```python
from build123d import *

# Parameters (mm, degrees)
SKETCH1_W                 = 100
SKETCH1_H                 = 155
BOSS_EXTRUDE1_DEPTH       = 7.5
SKETCH2_R                 = 2.05
SKETCH2_W                 = 60
SKETCH2_H                 = 17.5
HOLE_CUTOUTS_DEPTH        = 8.5
SKETCH3_W                 = 25
SKETCH3_H                 = 2.5
BATTERY_STRAP_HOLES_DEPTH = 8.5
H_BRIDGE_HOLES_DEPTH      = 7.5
FILLET1_R                 = 2
CAMERA_WIRE_HOLE_DEPTH    = 8.5
SKETCH10_R                = 2.05
CUT_EXTRUDE1_DEPTH        = 7.5
SKETCH11_R                = 3
CUT_EXTRUDE2_DEPTH        = 3


with BuildPart() as part:
    # Sketch1 → Boss-Extrude1 (new body)
    with BuildSketch(Plane.XY):
        with Locations((50, 77.5)):
            Rectangle(SKETCH1_W, SKETCH1_H)
    extrude(amount=BOSS_EXTRUDE1_DEPTH)

    # Sketch2 → Hole cutouts (cut, through all)
    with BuildSketch(Plane.XY.offset(7.5)):
        with Locations((10.45, 146.45)):
            Circle(SKETCH2_R)
        with Locations((89.95, 143.95)):
            Circle(SKETCH2_R)
        with Locations((89.95, 11.05)):
            Circle(SKETCH2_R)
        with Locations((10.45, 8.55)):
            Circle(SKETCH2_R)
        with Locations((50.2, 146.25)):
            Rectangle(SKETCH2_W, SKETCH2_H)
        with Locations((50.2, 8.75)):
            Rectangle(SKETCH2_W, SKETCH2_H)
    extrude(amount=-HOLE_CUTOUTS_DEPTH, mode=Mode.SUBTRACT)

    # Sketch3 → Battery strap holes (cut, through all)
    with BuildSketch(Plane.XY.offset(7.5)):
        with Locations((22.5, 89.75)):
            Rectangle(SKETCH3_W, SKETCH3_H)
        with Locations((77.5, 89.75)):
            Rectangle(SKETCH3_W, SKETCH3_H)
        with Locations((22.5, 55.25)):
            Rectangle(SKETCH3_W, SKETCH3_H)
        with Locations((77.5, 55.25)):
            Rectangle(SKETCH3_W, SKETCH3_H)
    extrude(amount=-BATTERY_STRAP_HOLES_DEPTH, mode=Mode.SUBTRACT)

    # Sketch4 → H-Bridge Holes (cut)
    with BuildSketch(Plane.XY.offset(7.5)):
        with BuildLine():
            Line((6, 133.51), (4, 133.51))
            ThreePointArc((4, 133.51), (2.25, 131.76), (4, 130.01))
            Line((4, 130.01), (5, 130.01))
            Line((5, 130.01), (5, 131.76))
            Line((5, 131.76), (7.75, 131.76))
            ThreePointArc((7.75, 131.76), (7.237436867, 132.997436867), (6, 133.51))
        make_face()
        with BuildLine():
            ThreePointArc((6, 130.01), (7.237436867, 130.522563133), (7.75, 131.76))
            Line((7.75, 131.76), (5, 131.76))
            Line((5, 131.76), (5, 130.01))
            Line((5, 130.01), (6, 130.01))
        make_face()
        with BuildLine():
            Line((42.5, 131.76), (39.75, 131.76))
            ThreePointArc((39.75, 131.76), (40.262563133, 130.522563133), (41.5, 130.01))
            Line((41.5, 130.01), (42.5, 130.01))
            Line((42.5, 130.01), (42.5, 131.76))
        make_face()
        with BuildLine():
            ThreePointArc((41.5, 133.51), (40.262563133, 132.997436867), (39.75, 131.76))
            Line((39.75, 131.76), (42.5, 131.76))
            Line((42.5, 131.76), (42.5, 130.01))
            Line((42.5, 130.01), (43.5, 130.01))
            ThreePointArc((43.5, 130.01), (45.25, 131.76), (43.5, 133.51))
            Line((43.5, 133.51), (41.5, 133.51))
        make_face()
        with BuildLine():
            Line((5, 94), (5, 95.75))
            Line((5, 95.75), (4, 95.75))
            ThreePointArc((4, 95.75), (2.25, 94), (4, 92.25))
            Line((4, 92.25), (6, 92.25))
            ThreePointArc((6, 92.25), (7.237436867, 92.762563133), (7.75, 94))
            Line((7.75, 94), (5, 94))
        make_face()
        with BuildLine():
            Line((6, 95.75), (5, 95.75))
            Line((5, 95.75), (5, 94))
            Line((5, 94), (7.75, 94))
            ThreePointArc((7.75, 94), (7.237436867, 95.237436867), (6, 95.75))
        make_face()
        with BuildLine():
            Line((43.5, 95.75), (42.5, 95.75))
            Line((42.5, 95.75), (42.5, 94))
            Line((42.5, 94), (39.75, 94))
            ThreePointArc((39.75, 94), (40.262563133, 92.762563133), (41.5, 92.25))
            Line((41.5, 92.25), (43.5, 92.25))
            ThreePointArc((43.5, 92.25), (45.25, 94), (43.5, 95.75))
        make_face()
        with BuildLine():
            Line((42.5, 94), (42.5, 95.75))
            Line((42.5, 95.75), (41.5, 95.75))
            ThreePointArc((41.5, 95.75), (40.262563133, 95.237436867), (39.75, 94))
            Line((39.75, 94), (42.5, 94))
        make_face()
    extrude(amount=-H_BRIDGE_HOLES_DEPTH, mode=Mode.SUBTRACT)

    # Fillet1
    fillet1_edges = [part.edges().sort_by_distance(p)[0] for p in [
        (20.2, 0, 3.75),
        (20.2, 17.5, 3.75),
        (80.2, 17.5, 3.75),
        (80.2, 0, 3.75),
        (20.2, 137.5, 3.75),
        (20.2, 155, 3.75),
        (80.2, 155, 3.75),
        (80.2, 137.5, 3.75),
        (0, 155, 3.75),
        (100, 155, 3.75),
        (100, 0, 3.75),
        (0, 0, 3.75),
    ]]
    fillet(fillet1_edges, radius=FILLET1_R)

    # Sketch9 → Camera Wire Hole (cut, through all)
    with BuildSketch(Plane.XY.offset(7.5)):
        with BuildLine():
            Line((0, 82.5), (0, 62.5))
            ThreePointArc((0, 62.5), (10, 72.5), (0, 82.5))
        make_face()
    extrude(amount=-CAMERA_WIRE_HOLE_DEPTH, mode=Mode.SUBTRACT)

    # Sketch10 → Cut-Extrude1 (cut)
    with BuildSketch(Plane.XY.offset(7.5)):
        with Locations((3.8, 4.55)):
            Circle(SKETCH10_R)
        with Locations((95.025, 42.825)):
            Circle(SKETCH10_R)
    extrude(amount=-CUT_EXTRUDE1_DEPTH, mode=Mode.SUBTRACT)

    # Sketch11 → Cut-Extrude2 (cut)
    with BuildSketch(Plane.XY.offset(7.5)):
        with Locations((3.8, 4.55)):
            Circle(SKETCH11_R)
        with Locations((95.025, 42.825)):
            Circle(SKETCH11_R)
        with BuildLine():
            Line((4, 97), (6, 97))
            ThreePointArc((6, 97), (9, 94), (6, 91))
            Line((6, 91), (4, 91))
            ThreePointArc((4, 91), (1, 94), (4, 97))
        make_face()
        with BuildLine():
            Line((41.5, 91), (43.5, 91))
            ThreePointArc((43.5, 91), (46.5, 94), (43.5, 97))
            Line((43.5, 97), (41.5, 97))
            ThreePointArc((41.5, 97), (38.5, 94), (41.5, 91))
        make_face()
        with BuildLine():
            Line((41.5, 128.5), (43.5, 128.5))
            ThreePointArc((43.5, 128.5), (46.5, 131.5), (43.5, 134.5))
            Line((43.5, 134.5), (41.5, 134.5))
            ThreePointArc((41.5, 134.5), (38.5, 131.5), (41.5, 128.5))
        make_face()
        with BuildLine():
            Line((4, 128.5), (6, 128.5))
            ThreePointArc((6, 128.5), (9, 131.5), (6, 134.5))
            Line((6, 134.5), (4, 134.5))
            ThreePointArc((4, 134.5), (1, 131.5), (4, 128.5))
        make_face()
    extrude(amount=-CUT_EXTRUDE2_DEPTH, mode=Mode.SUBTRACT)


solid = part.part
```
Check sheet for the modelled part. Datum: model origin and axes. Units: mm. A direction names the side the tool comes from. Give positions to 0.01 mm unless a question says otherwise; leave off trailing zeros. Loops run counter-clockwise (first coordinate to the right, second up) from the corner with the lowest first, then second, coordinate; pieces in that order, holes last. Notation, with made-up numbers: M -6,-7.5 L 11,-7.5 A17 ccw 11,22.5 Z; hole C 18,-31 d2. An arc over 180 degrees is marked long. Answer in a Markdown table with one row per item.
1) Mould release check, pull along X, two halves, no side actions. Record for faces 4 (the face through (80.2, 9, 4)), 5 (the face through (100, 76, 4)), 6 (the face through (50, 17.5, 4)), 7 (the face through (90, 155, 4)): released by +X, released by -X, zero draft, split by the parting line, or undercut.
Solutions:
| item | result |
|---|---|
| face 4 | undercut |
| face 5 | released by +X |
| face 6 | undercut |
| face 7 | zero draft |
2) Tool access check on faces 1 (the face through (50, 137.5, 4)), 2 (the face through (9, 94, 6)), 3 (the face through (2.25, 131.8, 2.28)). Record the directions out of +Z, -Z, +X, -X, +Y, -Y that give a thin tool (end or side, any length) a straight path to the whole face; none if there is none.
Solutions:
| item | result |
|---|---|
| face 1 | +Z, -Z, +Y |
| face 2 | +Z |
| face 3 | +Z, -Z |
3) Cross-section at A-A (x = 84). Enter the section's corners in (y, z), plus the area to 4 significant figures.
Solutions:
| item | result |
|---|---|
| outline | M 0,0 L 54,0 L 54,7.5 L 0,7.5 Z; M 56.5,0 L 88.5,0 L 88.5,7.5 L 56.5,7.5 Z; M 91,0 L 155,0 L 155,7.5 L 91,7.5 Z |
| area | 1,125 mm^2 |
4) Cross-section at B-B (y = 4.55). Enter the section's corners in (x, z), plus the area to 3 significant figures.
Solutions:
| item | result |
|---|---|
| outline | M 0,0 L 1.75,0 L 1.75,4.5 L 0.8,4.5 L 0.8,7.5 L 0,7.5 Z; M 5.85,0 L 20.2,0 L 20.2,7.5 L 6.8,7.5 L 6.8,4.5 L 5.85,4.5 Z; M 80.2,0 L 100,0 L 100,7.5 L 80.2,7.5 Z |
| area | 264 mm^2 |
5) Depth check by flat-ended pin: pin 1 (1 mm diameter, centred on x = 42.5, z = 3, fed in from +Y); pin 2 (1.8 mm diameter, centred on x = 4, y = 133, fed in from +Z); pin 3 (4 mm diameter, centred on x = 44, z = 3.5, fed in from -Y); pin 4 (1.8 mm diameter, centred on x = 41, y = 94.5, fed in from +Z). Enter the tip coordinate at first touch or a pass-through.
Solutions:
| item | result |
|---|---|
| pin 1 | stops at y = 137.5 |
| pin 2 | stops at z = 4.5 |
| pin 3 | stops at y = 17.5 |
| pin 4 | passes through |
6) Thickness scan on line 1 (Y direction, x = 10.45, z = 5.5); line 2 (X direction, y = 143.95, z = 2); line 3 (X direction, y = 55.5, z = 4.25). Record the ranges inside material, lowest first.
Solutions:
| item | result |
|---|---|
| line 1 | y = 0 to 6.5, 10.6 to 54, 56.5 to 88.5, 91 to 144.4, 148.5 to 155 |
| line 2 | x = 0 to 20.2, 80.2 to 87.9, 92 to 100 |
| line 3 | x = 0 to 10, 35 to 65, 90 to 100 |
7) Cross-section at C-C (x = 71). Enter the section's corners in (y, z).
Solutions:
| item | result |
|---|---|
| outline | M 17.5,0 L 54,0 L 54,7.5 L 17.5,7.5 Z; M 56.5,0 L 88.5,0 L 88.5,7.5 L 56.5,7.5 Z; M 91,0 L 137.5,0 L 137.5,7.5 L 91,7.5 Z |
